Design review of the part built by this model. Coordinates are the model's own, in mm. A direction names the side the tool comes from. Coordinates: 2 decimals unless noted, no trailing zeros. Write each loop counter-clockwise with the first axis right and the second up, starting at its lowest first coordinate (ties: lowest second). Pieces come first, ordered by that corner, then holes. Notation, with made-up numbers: (62.25, 18.5) -> (87.25, 18.5) arc R25 ccw to (87.25, 51.5) -> close; hole circle Ø5 at (-37, 59.25). An arc over 180 degrees is marked (long way). Answer in a Markdown table with one row per item. Add a question column.
Item 1: Take a section at A-A, the plane z = 0. Write out the cut boundary in (x, y).
Item 2: Take a section at B-B, the plane x = 0. Write out the cut boundary in (y, z), and give its area (3 significant figures).
Item 3: To check wall thickness, follow line 1 (Y direction, x = -3, z = -6.25); line 2 (X direction, y = 2.5, z = 3); line 3 (X direction, y = 1.5, z = -4). State the ranges of each line that lie inside material, in increasing order.
Item 4: Take a section at C-C, the plane y = 0.5. Write out the cut boundary in (x, z), and give its area (3 significant figures).
Item 5: For faces 5 (the face through (6.35, 4, 0)), 6 (the face through (0, 2, -7)), 7 (the face through (0, 6, 0)), list the 3-axis set-ups (+Z, -Z, +X, -X, +Y, -Y) from which the entire face can be reached by the end or side of a thin tool; tool diameter is ignored.
Item 6: Take a section at D-D, the plane y = 4.5. Write out the cut boundary in (x, z) (3 decimals).
Item 7: Draft analysis for pull direction Z (two halves, no side actions). For faces 1 (the face through (7, 3.3, 0)), 2 (the face through (-1.07, 2.79, 8.18)), 3 (the face through (0, 1, -6)), 4 (the face through (7, 4, -0.975)), state which applies: released by +Z, released by -Z, zero draft, split by the parting line, or undercut.
Item 8: Clearance check with flat-ended pins moving along their axes: P1, Ø2, axis at x = 7, y = 4, coming from the +Z side; P2, Ø1.5, axis at y = 1.5, z = 3.5, coming from the +X side; P3, Ø1, axis at x = -2.5, y = 4.5, coming from the +Z side. State where each tip first meets the part, or that it passes through.
from build123d import *

# Parameters (mm, degrees)
SKETCH100_W     = 14
SKETCH100_H     = 2
PAD063_DEPTH    = 3
SKETCH110_R     = 8.25
PAD067_DEPTH    = 6
POCKET022_DEPTH = 2.7
FILLET009_R     = 0.5


with BuildPart() as hole006:
    # Sketch100 → Pad063 (new body)
    with BuildSketch(Plane.XY):
        with Locations((0, 1)):
            Rectangle(SKETCH100_W, SKETCH100_H)
    extrude(amount=PAD063_DEPTH)


with BuildPart() as hole006_1:
    # Body025 placement: moved
    add(hole006.part.moved(Location((0, 0, -9))))


with BuildPart() as metal_case001:
    # Sketch110 → Pad067 (new body)
    with BuildSketch(Plane.XZ):
        Circle(SKETCH110_R)
    extrude(amount=PAD067_DEPTH)

    # Sketch102 (on Face2 of Pad067) → Pocket022 (cut)
    with BuildSketch(Plane(origin=(0, 0, 0), x_dir=(1, 0, 0), z_dir=(0, 1, 0))):
        Polygon((6.35, 0.975), (8.25, 0.975), (8.25, -0.975), (6.35, -0.975), (6.35, 0), align=None)
    extrude(amount=-POCKET022_DEPTH, mode=Mode.SUBTRACT)

    # Fillet009
    fillet009_edges = [metal_case001.edges().sort_by_distance(p)[0] for p in [
        (7.271092, 0, 0.975),
        (6.35, 0, 0.4875),
        (6.35, 0, -0.4875),
        (7.271092, 0, -0.975),
        (-8.25, 0, 0),
    ]]
    fillet(fillet009_edges, radius=FILLET009_R)


with BuildPart() as metal_case001_1:
    # Body027 placement: moved
    add(metal_case001.part.moved(Location((0, 6, 0))))

    # Cut001: cut Hole006
    add(hole006_1.part, mode=Mode.SUBTRACT)


solid = metal_case001_1.part
Answers:
| question | item | result |
|---|---|---|
| 1 | outline | (-8.25, 0) -> (8.25, 0) -> (8.25, 3.3) -> (6.35, 3.3) -> (6.35, 5.5) arc R0.5 ccw to (5.85, 6) -> (-7.75, 6) arc R0.5 ccw to (-8.25, 5.5) -> close |
| 2 | outline | (0, -6) -> (2, -6) -> (2, -8.25) -> (5.5, -8.25) arc R0.5 ccw to (6, -7.75) -> (6, 7.75) arc R0.5 ccw to (5.5, 8.25) -> (0, 8.25) -> close |
| 2 | area | 94.4 mm^2 |
| 3 | line 1 | y = 2 to 6 |
| 3 | line 2 | x = -7.69 to 7.69 |
| 3 | line 3 | x = -7.22 to 7.22 |
| 4 | outline | (-5.66, -6) -> (5.66, -6) arc R8.25 ccw (long way) to start |
| 4 | area | 196 mm^2 |
| 5 | face 5 | +X, +Y |
| 5 | face 6 | -Z, +X, -X, -Y |
| 5 | face 7 | +Z, -Z, +X, -X, +Y |
| 6 | outline | (6.35, -0.975) -> (6.35, 0.975) -> (8.192, 0.975) arc R8.25 ccw (long way) to (8.192, -0.975) -> close |
| 7 | face 1 | undercut |
| 7 | face 2 | split by the parting line |
| 7 | face 3 | released by -Z |
| 7 | face 4 | undercut |
| 8 | P1 | stops at z = 5.66 |
| 8 | P2 | stops at x = 7.78 |
| 8 | P3 | stops at z = 8 |
